Answer from the drawing. Dimensions are ordinates in mm from the lowest x, y and z of the part. A direction names the side the tool comes from. Round coordinates to 2 decimals unless told otherwise and drop trailing zeros. Write each loop counter-clockwise with the first axis right and the second up, starting at its lowest first coordinate (ties: lowest second). Pieces come first, ordered by that corner, then holes.
1. Find section B-B (z = 5). Write down the section's boundary in (x, y), and give its area (3 significant figures).
2. Flat-ended cylindrical pins translate along their axes: pin 1 Ø1.5 at (x, z) = (3, 5) entering from -Y; pin 2 Ø6 at (x, y) = (5, 4) entering from -Z; pin 3 Ø3 at (y, z) = (3, 7.5) entering from -X; pin 4 Ø1.5 at (y, z) = (7, 7.5) entering from -X. Find the tip coordinate at first contact, or state that the pin passes through.
3. Straight lines are drawn through the part: probe 1 along X at (y, z) = (1.75, 5); probe 2 along X at (y, z) = (2.5, 2.25); probe 3 along Y at (x, z) = (7, 2.5). For each, find the intervals that lie inside material, in ascending order.
4. Find section A-A (x = 5). Write down the section's boundary in (y, z), and give its area (3 significant figures).
5. A tool of negligible diameter and unlimited length cuts with its end or side. For the marked faces 4 and 5, from which of +Z, -Z, +X, -X, +Y, -Y can it reach the whole face along a straight path? Write none if from no direction.
6. Find section C-C (y = 5.5). Write down the section's boundary in (x, z), and give its area (3 significant figures).
7. Determine the mould class of the marked faces 1, 2 and 3 for opening direction Y: pulls with the +Y half, pulls with the -Y half, needs draft (parallel to the pull), parting line crosses it, or undercut.
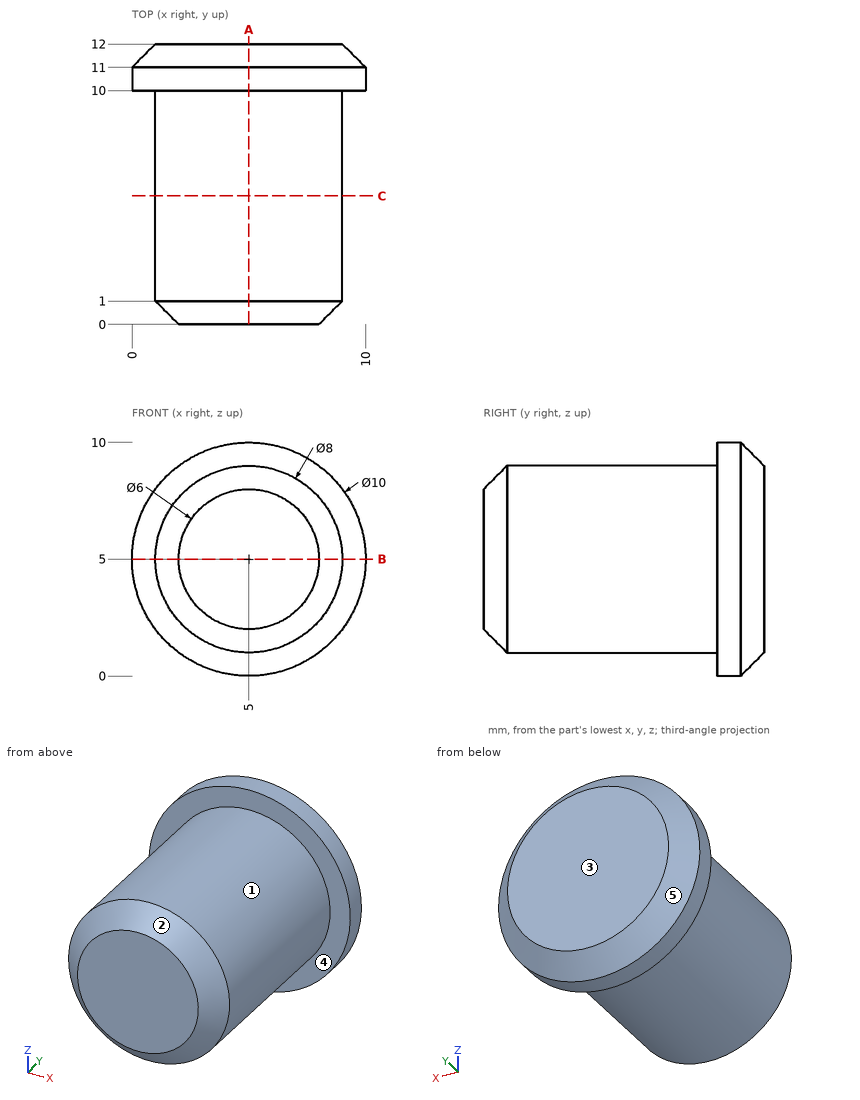
Worked answers:
1. outline: (0, 10) - (1, 10) - (1, 1) - (2, 0) - (8, 0) - (9, 1) - (9, 10) - (10, 10) - (10, 11) - (9, 12) - (1, 12) - (0, 11) - close
1. area: 98.0 mm2
2. pin 1: stops at y = 0
2. pin 2: stops at z = 1
2. pin 3: stops at x = 1.13
2. pin 4: stops at x = 1.4
3. probe 1: x = 1 to 9
3. probe 2: x = 2.1 to 7.9
3. probe 3: y = 0.2 to 12
4. outline: (0, 2) - (1, 1) - (10, 1) - (10, 0) - (11, 0) - (12, 1) - (12, 9) - (11, 10) - (10, 10) - (10, 9) - (1, 9) - (0, 8) - close
4. area: 98.0 mm2
5. face 4: -Y
5. face 5: +Y
6. outline: circle Ø8 at (5, 5)
6. area: 50.3 mm2
7. face 1: needs draft
7. face 2: pulls with the -Y half
7. face 3: pulls with the +Y half
